Check sheet for the modelled part. Datum: model origin and axes. Units: mm. A direction names the side the tool comes from. Coordinates: 2 decimals unless noted, no trailing zeros. Loops run counter-clockwise (first coordinate to the right, second up) from the corner with the lowest first, then second, coordinate; pieces in that order, holes last. Notation, with made-up numbers: M 56.5,4.25 L 69.5,4.25 A4 ccw 69.5,8.25 Z; hole C 31,58 d11. An arc over 180 degrees is marked long. Return JSON: item names as keys, results as strings.
from build123d import *

# Parameters (mm, degrees)
BOSS_EXTRUDE2_DEPTH                  = 26.75
BOSS_EXTRUDE2_DEPTH_BACK             = 26.75
SKETCH3_R                            = 1.5
TOP_FORM_DEPTH                       = 108.569617744
TOP_FORM_DEPTH_BACK                  = 108.569617744
SKETCH12_OUTSIDE_W                   = 131.712
SKETCH12_OUTSIDE_H                   = 79.73
END_EXTRUDE_DEPTH                    = 26.75
END_EXTRUDE_DEPTH_BACK               = 26.75
SKETCH13_R                           = 1.5
SPRING_PHALANX_PLACE_DEPTH           = 8.038475773
SPRING_SUPPORT_DEPTH                 = 3
SPRING_SUPPORT_CORNER_CUT_DEPTH      = 108.569617744
SPRING_SUPPORT_CORNER_CUT_DEPTH_BACK = 108.569617744
SPRING_PLACE_CUT_DEPTH               = 17.5
SPRING_PLACE_CUT_DEPTH_BACK          = 17.5
PHALANX_SPACE_CUT_DEPTH              = 108.487219822
PHALANX_SPACE_CUT_DEPTH_BACK         = 108.487219822


with BuildPart() as part:
    # Sketch3 → Boss-Extrude2 (new, two sides: drawn at the far end of the back side and taken through both)
    with BuildSketch(Plane.XY.offset(-BOSS_EXTRUDE2_DEPTH_BACK)):
        with BuildLine():
            Line((0.970571419, 3.622221849), (-69.482255776, 22.5))
            Line((-69.482255776, 22.5), (-79.701126542, 22.5))
            Line((-79.701126542, 22.5), (-96.234008051, 14.790590741))
            Line((-96.234008051, 14.790590741), (-101.732050808, 3))
            Line((-101.732050808, 3), (-100, 0))
            Line((-100, 0), (-74.714962449, 14.598323237))
            Line((-74.714962449, 14.598323237), (-68.970571419, 14.598323237))
            Line((-68.970571419, 14.598323237), (-0.970571419, -3.622221849))
            ThreePointArc((-0.970571419, -3.622221849), (3.622221849, -0.970571419), (0.970571419, 3.622221849))
        make_face()
        Circle(SKETCH3_R, mode=Mode.SUBTRACT)
    extrude(amount=BOSS_EXTRUDE2_DEPTH + BOSS_EXTRUDE2_DEPTH_BACK)

    # Sketch12 outside → top-form (cut, two sides: drawn at the far end of the back side and taken through both)
    with BuildSketch(Plane(origin=(0, 0, 0), x_dir=(1, 0, 0), z_dir=(0, 1, 0)).offset(-TOP_FORM_DEPTH_BACK)):
        with Locations((-48.991, 0)):
            Rectangle(SKETCH12_OUTSIDE_W, SKETCH12_OUTSIDE_H)
        Polygon((-101.732050808, 10), (-101.732050808, -10), (-18.75, -20), (-3.75, -26.75), (-3.75, 26.75), (-18.75, 20), align=None, mode=Mode.SUBTRACT)
    extrude(amount=TOP_FORM_DEPTH + TOP_FORM_DEPTH_BACK, mode=Mode.SUBTRACT)

    # Sketch13 → end-extrude (add, two sides: drawn at the far end of the back side and taken through both)
    with BuildSketch(Plane.XY.offset(-END_EXTRUDE_DEPTH_BACK)):
        with BuildLine():
            Line((-3.75, 4.887095148), (-3.75, -2.877476205))
            Line((-3.75, -2.877476205), (-0.970571419, -3.622221849))
            ThreePointArc((-0.970571419, -3.622221849), (3.622221849, -0.970571419), (0.970571419, 3.622221849))
            Line((0.970571419, 3.622221849), (-3.75, 4.887095148))
        make_face()
        Circle(SKETCH13_R, mode=Mode.SUBTRACT)
    extrude(amount=END_EXTRUDE_DEPTH + END_EXTRUDE_DEPTH_BACK)

    # Sketch16 → spring_phalanx_place (cut, along a direction that is not the sketch's normal)
    with BuildSketch(Plane(origin=(0.970571419, 3.622221849, 0), x_dir=(0.9659258262890683, -0.2588190451025211, 0), z_dir=(0.2588190451025211, 0.9659258262890683, 0))):
        Polygon((-4.887095148, 0), (-4.887095148, -21.75), (0, -21.75), (0, 21.75), (-4.887095148, 21.75), align=None)
        Polygon((0, 21.75), (0, -21.75), (3.75, -21.75), (3.75, 0), (3.75, 21.75), align=None)
    extrude(amount=-SPRING_PHALANX_PLACE_DEPTH, dir=(0, 1, 0), mode=Mode.SUBTRACT)

    # spikes cone 1 section (through the dimple's axis) → spikes (revolve)
    with BuildSketch(Plane(origin=(-98.700961894, 0.75, 8.857123826), x_dir=(0, 0, 1), z_dir=(0.866025404, 0.5, 0))):
        Polygon((0, 0), (0.75, 0), (0, 3.528472582), align=None)
    revolve(axis=Axis((-98.700961894, 0.75, 8.857123826), (0.5, -0.866025404, 0)))

    # spikes cone 2 section (through the dimple's axis) → spikes cone 2 (revolve)
    with BuildSketch(Plane(origin=(-98.700961894, 0.75, -8.857123826), x_dir=(0, 0, 1), z_dir=(0.866025404, 0.5, 0))):
        Polygon((0, 0), (0.75, 0), (0, 3.528472582), align=None)
    revolve(axis=Axis((-98.700961894, 0.75, -8.857123826), (0.5, -0.866025404, 0)))

    # Sketch18 → spring-support (add)
    with BuildSketch(Plane(origin=(-0.970571419, -3.622221849, 0), x_dir=(0.9659258262890681, -0.2588190451025214, 0), z_dir=(-0.2588190451025214, -0.9659258262890681, 0))):
        Polygon((-2.877476205, 21.75), (-2.877476205, 26.75), (-18.406618911, 20), (-18.406618911, -20), (-2.877476205, -26.75), (-2.877476205, -21.75), align=None)
    extrude(amount=SPRING_SUPPORT_DEPTH)

    # Sketch22 → spring-support-corner-cut (cut, two sides: drawn at the far end of the back side and taken through both)
    with BuildSketch(Plane.XY.offset(-SPRING_SUPPORT_CORNER_CUT_DEPTH_BACK)):
        Polygon((-19.526457135, -1.756015797), (-18.75, 1.141761682), (-12.026457135, -3.765634741), align=None)
    extrude(amount=SPRING_SUPPORT_CORNER_CUT_DEPTH + SPRING_SUPPORT_CORNER_CUT_DEPTH_BACK, mode=Mode.SUBTRACT)

    # Sketch22<3> → spring-place-cut (cut, two sides: drawn at the far end of the back side and taken through both)
    with BuildSketch(Plane.XY.offset(-SPRING_PLACE_CUT_DEPTH_BACK)):
        Polygon((-3.75, -1.842200025), (-10.994443697, 0.098942814), (-8.406253246, 9.758201077), (-3.75, 8.51056178), align=None)
    extrude(amount=SPRING_PLACE_CUT_DEPTH + SPRING_PLACE_CUT_DEPTH_BACK, mode=Mode.SUBTRACT)

    # Sketch21 → phalanx-space-cut (cut, two sides: drawn at the far end of the back side and taken through both)
    with BuildSketch(Plane(origin=(-0.711752374, -2.656296022, 0), x_dir=(0.9659258262890681, -0.2588190451025214, 0), z_dir=(0.2588190451025214, 0.9659258262890681, 0)).offset(-PHALANX_SPACE_CUT_DEPTH_BACK)):
        Polygon((-4.887095148, 21.75), (0, 21.75), (0, 16.25), (-5, 16.25), (-5, 21.75), align=None)
        Polygon((-4.887095148, -21.75), (-5, -21.75), (-5, -16.25), (0, -16.25), (0, -21.75), align=None)
    extrude(amount=PHALANX_SPACE_CUT_DEPTH + PHALANX_SPACE_CUT_DEPTH_BACK, mode=Mode.SUBTRACT)


solid = part.part
1) Draft check along X on faces 5 (the face through (-59.66, 13.59, -15.07)), 6 (the face through (-10.165, 3.194, -0.245)), 7 (the face through (-4.133, -4.306, -24.285)). Enter one of: +X half, -X half, draft (parallel to the pull), parting line (faces both ways), or undercut.
Answers:
{"face 5": "-X half", "face 6": "+X half", "face 7": "undercut"}
2) Go/stop test with flat-tipped pins: pin 1 Ø4.5 at (x, z) = (-72, 4) entering from -Y; pin 2 Ø1.5 at (y, z) = (9, -21.5) entering from +X; pin 3 Ø0.8 at (x, y) = (-5, -3.5) entering from -Z; pin 4 Ø1.4 at (x, y) = (-5.5, -3.5) entering from +Z. Record where each tip stops, or that it passes through.
Answers:
{"pin 1": "y = 14.6", "pin 2": "through", "pin 3": "z = -26.47", "pin 4": "z = 26.39"}
3) Section check B-B on x = -77. Record the cut outline in (y, z), then the cut area to 3 significant figures.
Answers:
{"outline": "M 13.28,-12.98 L 22.5,-12.98 L 22.5,12.98 L 13.28,12.98 Z", "area": "239 mm²"}
4) Section check A-A on z = 3.5. Record the cut outline in (x, y).
Answers:
{"outline": "M -101.73,3 L -100,0 L -74.71,14.6 L -68.97,14.6 L -18.75,1.14 L -12.03,-3.77 L -4.53,-5.78 L -3.75,-2.88 L -3.75,-1.84 L -10.99,0.1 L -9.31,6.38 L -69.48,22.5 L -79.7,22.5 L -96.23,14.79 Z"}
5) Section check C-C on x = -59.5. Record the cut outline in (y, z).
Answers:
{"outline": "M 12.06,-15.09 L 19.83,-15.09 L 19.83,15.09 L 12.06,15.09 Z"}
6) Scan lines: line 1 along Y through (x, z) = (0, 24.6); line 2 along X through (y, z) = (0, -24.15); line 3 along Z through (x, y) = (-66.5, 14). Record each from-to range of solid material in increasing order. Write a range as [from, to].
Answers:
{"line 1": "[-3.75, -1.5], [1.5, 3.88]", "line 2": "[-9.53, -1.5], [1.5, 3.75]", "line 3": "[-14.25, 14.25]"}
7) Set-up check for faces 1 (the face through (-2, 0, -21.75)), 2 (the face through (-2.38, -3.245, -24.285)), 3 (the face through (-7, 3, 17.5)), 4 (the face through (-98.945, 8.978, -0.149)): record each of +Z, -Z, +X, -X, +Y, -Y from which the full face is reachable in a straight line by a thin tool's end or side.
Answers:
{"face 1": "+X, -Y", "face 2": "+Z, -Z, -Y", "face 3": "+X", "face 4": "+Z, -Z, -X, +Y"}
